Read the model definition and answer for the solid it produces. Units are mm, in the model's axes. Face numbers are marked on the shaded views. A direction names the side the tool comes from. Coordinates: 2 decimals unless noted, no trailing zeros. Loops run counter-clockwise (first coordinate to the right, second up) from the corner with the lowest first, then second, coordinate; pieces in that order, holes last. Notation, with made-up numbers: (25.5, 34) -> (39.5, 34) arc R12 ccw to (39.5, 55) -> close; hole circle Ø1 at (77.25, 55.5). An arc over 180 degrees is marked (long way). Answer as CSV lines item,"result".
Autodesk Inventor part; units mm, degrees
ref_plane "YZ Plane" through (0, 0, 0) normal (1, 0, 0) x (0, 1, 0)
ref_plane "XZ Plane" through (0, 0, 0) normal (0, 1, 0) x (-1, 0, 0)
ref_plane "XY Plane" through (0, 0, 0) normal (0, 0, 1) x (1, 0, 0)
sketch "Sketch1" plane through (0, 0, 0) normal (0, 0, 1) x (1, 0, 0)
  line L0 (-21.1, 29.81) -> (21.1, 29.81)
  line L1 (21.1, 29.81) -> (21.1, -29.81)
  line L2 (21.1, -29.81) -> (-21.1, -29.81)
  line L3 (-21.1, -29.81) -> (-21.1, 29.81)
  line L4 (0, 0) -> (0, 68.2086)
  line L5 (0, 0) -> (53.7664, 0)
  line L6 (-21.1, 29.81) -> (21.1, 29.81)
  line L7 (21.1, 29.81) -> (21.1, -29.81)
  line L8 (21.1, -29.81) -> (-21.1, -29.81)
  line L9 (-21.1, -29.81) -> (-21.1, 29.81)
  line L10 (0, 0) -> (0, 68.2086)
  line L11 (0, 0) -> (54.462, 0)
  line L12 (-23.1, 31.81) -> (23.1, 31.81)
  line L13 (23.1, 31.81) -> (23.1, -31.81)
  line L14 (23.1, -31.81) -> (-23.1, -31.81)
  line L15 (-23.1, -31.81) -> (-23.1, 31.81)
  line L16 (-26.1, 34.81) -> (26.1, 34.81)
  line L17 (26.1, 34.81) -> (26.1, -34.81)
  line L18 (26.1, -34.81) -> (-26.1, -34.81)
  line L19 (-26.1, -34.81) -> (-26.1, 34.81)
  dimension "d0" = 59.62
  dimension "d1" = 42.2
  dimension "d2" = 59.62
  dimension "d3" = 42.2
  dimension "d4" = 2
  dimension "d5" = 2
  dimension "d6" = 0
  dimension "d7" = 3
  dimension "d8" = 3
extrude "Extrusion1" add sketch "Sketch1" along normal blind 30.3 contours L3 L2 L1 L5 L13 L14 L15 L12 L4 L0 | L4 L12 L13 L5 L1 L0
sketch "Sketch2" plane through (0, 0, 30.3) normal (0, 0, 1) x (1, 0, 0)
  line L0 (-23.1, -31.81) -> (23.1, -31.81)
  line L1 (23.1, -31.81) -> (23.1, 31.81)
  line L2 (23.1, 31.81) -> (-23.1, 31.81)
  line L3 (-23.1, 31.81) -> (-23.1, -31.81)
  point P0 (0, 0)
extrude "Extrusion2" add sketch "Sketch2" along normal blind 2
sketch "Sketch3" plane through (0, 0, 0) normal (0, 0, -1) x (-1, 0, 0)
  line L0 (-23.1, -31.81) -> (23.1, -31.81)
  line L1 (23.1, -31.81) -> (23.1, 31.81)
  line L2 (23.1, 31.81) -> (-23.1, 31.81)
  line L3 (-23.1, 31.81) -> (-23.1, -31.81)
  circle A0 centre (-3.92, 14.54) radius 10.07
  line L4 (21.1, 29.81) -> (21.1, -29.81)
  line L5 (-21.1, 29.81) -> (21.1, 29.81)
  line L6 (-21.1, -29.81) -> (-21.1, 29.81)
  line L7 (21.1, -29.81) -> (-21.1, -29.81)
  point P0 (0, 0)
  point P1 (0, 0)
extrude "Extrusion3" add sketch "Sketch3" along normal blind 2 contours L3 L2 L1 L0 | L4 L7 L6 L5
fillet "Fillet3" radius 3 4 edges at (-23.1, -31.81, 15.15) (-23.1, 31.81, 15.15) (23.1, -31.81, 15.15) (23.1, 31.81, 15.15)
equation "\"d5\" = d4"
equation "\"d8\" = d7"
properties part number "Cam.Silicon.back" material "Silicone"
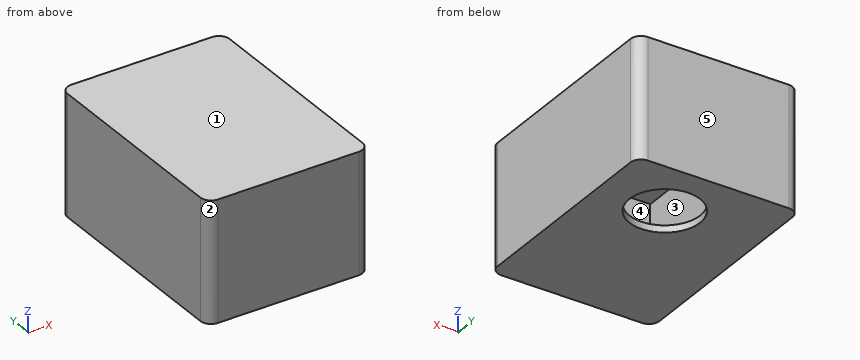
Q1. Find the intervals of material crossed by probe 1 along X at (y, z) = (8, 11); probe 2 along Y at (x, z) = (-11, 30); probe 3 along Z at (x, y) = (-6.5, 26), in increasing order. Write a range as [from, to].
Results:
probe 1,"x = [-23.1, -21.1], [21.1, 23.1]"
probe 2,"y = [-31.81, -29.81], [29.81, 31.81]"
probe 3,"z = [-2, 0], [30.3, 32.3]"
Q2. A cutting plane is placed at A-A, the plane z = 9.5. Write down the section's boundary in (x, y).
Results:
outline,"(-23.1, -28.81) arc R3 ccw to (-20.1, -31.81) -> (20.1, -31.81) arc R3 ccw to (23.1, -28.81) -> (23.1, 28.81) arc R3 ccw to (20.1, 31.81) -> (-20.1, 31.81) arc R3 ccw to (-23.1, 28.81) -> close; hole (-21.1, -29.81) -> (21.1, -29.81) -> (21.1, 29.81) -> (-21.1, 29.81) -> close"
Q3. Given pin 1 Ø18 at (x, y) = (3.92, 14.54) entering from -Z, flat-ended and moving along its own axis, determine where the tip first touches the part or whether it passes through.
Results:
pin 1,"stops at z = 30.3"
Q4. A cutting plane is placed at D-D, the plane y = -12. Write down the section's boundary in (x, z).
Results:
outline,"(-23.1, -2) -> (23.1, -2) -> (23.1, 32.3) -> (-23.1, 32.3) -> close; hole (-21.1, 0) -> (21.1, 0) -> (21.1, 30.3) -> (-21.1, 30.3) -> close"
Q5. A cutting plane is placed at C-C, the plane y = 14.54. Write down the section's boundary in (x, z), and give its area (3 significant figures).
Results:
outline,"(-23.1, -2) -> (-6.15, -2) -> (-6.15, 0) -> (-21.1, 0) -> (-21.1, 30.3) -> (21.1, 30.3) -> (21.1, 0) -> (13.99, 0) -> (13.99, -2) -> (23.1, -2) -> (23.1, 32.3) -> (-23.1, 32.3) -> close"
area,"266 mm²"
Q6. For the marked faces 4 and 5, determine the directions among +Z, -Z, +X, -X, +Y, -Y from which every point of the face is accessible in a straight line to the end or side of a thin tool.
Results:
face 4,"none"
face 5,"+Z, -Z, +X, -X, +Y"
Q7. For a pull along Z with two mould halves and no side action, classify the marked faces 1, 2 and 3 as pulls with the +Z half, pulls with the -Z half, needs draft (parallel to the pull), parting line crosses it, or undercut.
Results:
face 1,"pulls with the +Z half"
face 2,"needs draft"
face 3,"undercut"
Q8. A cutting plane is placed at B-B, the plane x = 17.5. Write down the section's boundary in (y, z), and give its area (3 significant figures).
Results:
outline,"(-31.81, -2) -> (31.81, -2) -> (31.81, 32.3) -> (-31.81, 32.3) -> close; hole (-29.81, 0) -> (29.81, 0) -> (29.81, 30.3) -> (-29.81, 30.3) -> close"
area,"376 mm²"
